```python
from build123d import *

# Parameters (mm, degrees)
SKETCH1_R           = 1.435
SKETCH1_R_2         = 1.4351
BOSS_EXTRUDE1_DEPTH = 3.175
SKETCH2_W           = 368.3
SKETCH2_H           = 127
CUT_EXTRUDE1_DEPTH  = 342.698968356
SKETCH4_R           = 1.89865
CUT_EXTRUDE2_DEPTH  = 342.698968356
SKETCH5_R           = 1.89865
CUT_EXTRUDE3_DEPTH  = 342.698968356


with BuildPart() as part:
    # Sketch1 → Boss-Extrude1 (new body)
    with BuildSketch(Plane.XY):
        with BuildLine():
            ThreePointArc((2.968751211, -181.189695026), (41.295889155, -181.079537948), (79.6220041, -180.778621425))
            Line((79.6220041, -180.778621425), (85.559165015, -180.714940362))
            ThreePointArc((85.559165015, -180.714940362), (123.887667874, -180.193645916), (162.213100977, -179.481566675))
            ThreePointArc((162.213100977, -179.481566675), (165.18118139, -179.418457741), (168.149237253, -179.35420455))
            ThreePointArc((168.149237253, -179.35420455), (192.659124698, -178.779845314), (217.167059321, -178.127456184))
            ThreePointArc((217.167059321, -178.127456184), (220.135246662, -178.043143258), (223.103401271, -177.957685792))
            Line((223.103401271, -177.957685792), (258.423629847, -176.852835003))
            ThreePointArc((258.423629847, -176.852835003), (267.290868319, -175.133004675), (275.18450496, -170.742533734))
            ThreePointArc((275.18450496, -170.742533734), (277.610750544, -168.6061656), (279.781359306, -166.210504095))
            ThreePointArc((279.781359306, -166.210504095), (284.283709644, -158.379432473), (286.129131597, -149.53685032))
            ThreePointArc((286.129131597, -149.53685032), (287.482131945, -117.828809116), (288.512976487, -86.108660213))
            ThreePointArc((288.512976487, -86.108660213), (288.592974065, -83.139049998), (288.670148028, -80.169365063))
            ThreePointArc((288.670148028, -80.169365063), (289.416235277, -41.572865854), (289.685382101, -2.970094485))
            ThreePointArc((289.685382101, -2.970094485), (289.686328933, 0.0005929), (289.684451162, 2.971279842))
            ThreePointArc((289.684451162, 2.971279842), (289.409759592, 41.084465923), (288.670148028, 79.191465063))
            ThreePointArc((288.670148028, 79.191465063), (288.592974065, 82.161149998), (288.512976487, 85.130760213))
            ThreePointArc((288.512976487, 85.130760213), (287.482131945, 116.850909116), (286.129131597, 148.55895032))
            ThreePointArc((286.129131597, 148.55895032), (284.283709644, 157.401532473), (279.781359306, 165.232604095))
            ThreePointArc((279.781359306, 165.232604095), (277.610750544, 167.6282656), (275.18450496, 169.764633734))
            ThreePointArc((275.18450496, 169.764633734), (267.290868319, 174.155104675), (258.423629847, 175.874935003))
            ThreePointArc((258.423629847, 175.874935003), (240.76414932, 176.447620699), (223.103401271, 176.979785792))
            ThreePointArc((223.103401271, 176.979785792), (220.135246662, 177.065243258), (217.167059321, 177.149556184))
            ThreePointArc((217.167059321, 177.149556184), (192.659124698, 177.801945314), (168.149237253, 178.37630455))
            ThreePointArc((168.149237253, 178.37630455), (165.18118139, 178.440557741), (162.213100977, 178.503666675))
            ThreePointArc((162.213100977, 178.503666675), (123.887667874, 179.215745916), (85.559165015, 179.737040362))
            ThreePointArc((85.559165015, 179.737040362), (82.590590695, 179.769453121), (79.6220041, 179.800721425))
            ThreePointArc((79.6220041, 179.800721425), (41.295889155, 180.101637948), (2.968751211, 180.211795026))
            ThreePointArc((2.968751211, 180.211795026), (0, 180.212367286), (-2.968751211, 180.211795026))
            ThreePointArc((-2.968751211, 180.211795026), (-41.295889155, 180.101637948), (-79.6220041, 179.800721425))
            ThreePointArc((-79.6220041, 179.800721425), (-82.590590695, 179.769453121), (-85.559165015, 179.737040362))
            ThreePointArc((-85.559165015, 179.737040362), (-123.887667874, 179.215745916), (-162.213100977, 178.503666675))
            ThreePointArc((-162.213100977, 178.503666675), (-165.18118139, 178.440557741), (-168.149237253, 178.37630455))
            ThreePointArc((-168.149237253, 178.37630455), (-192.659124698, 177.801945314), (-217.167059321, 177.149556184))
            ThreePointArc((-217.167059321, 177.149556184), (-220.135246662, 177.065243258), (-223.103401271, 176.979785792))
            ThreePointArc((-223.103401271, 176.979785792), (-240.76414932, 176.447620699), (-258.423629847, 175.874935003))
            ThreePointArc((-258.423629847, 175.874935003), (-267.290868319, 174.155104675), (-275.18450496, 169.764633734))
            ThreePointArc((-275.18450496, 169.764633734), (-277.610750544, 167.6282656), (-279.781359306, 165.232604095))
            ThreePointArc((-279.781359306, 165.232604095), (-284.283709644, 157.401532473), (-286.129131597, 148.55895032))
            ThreePointArc((-286.129131597, 148.55895032), (-287.482131945, 116.850909116), (-288.512976487, 85.130760213))
            ThreePointArc((-288.512976487, 85.130760213), (-288.592974065, 82.161149998), (-288.670148028, 79.191465063))
            ThreePointArc((-288.670148028, 79.191465063), (-289.409759592, 41.084465923), (-289.684451162, 2.971279842))
            ThreePointArc((-289.684451162, 2.971279842), (-289.686328933, 0.0005929), (-289.685382101, -2.970094485))
            ThreePointArc((-289.685382101, -2.970094485), (-289.416235277, -41.572865854), (-288.670148028, -80.169365063))
            ThreePointArc((-288.670148028, -80.169365063), (-288.592974065, -83.139049998), (-288.512976487, -86.108660213))
            ThreePointArc((-288.512976487, -86.108660213), (-287.482131945, -117.828809116), (-286.129131597, -149.53685032))
            ThreePointArc((-286.129131597, -149.53685032), (-284.283709644, -158.379432473), (-279.781359306, -166.210504095))
            ThreePointArc((-279.781359306, -166.210504095), (-277.610750544, -168.6061656), (-275.18450496, -170.742533734))
            ThreePointArc((-275.18450496, -170.742533734), (-267.290868319, -175.133004675), (-258.423629847, -176.852835003))
            ThreePointArc((-258.423629847, -176.852835003), (-240.76414932, -177.425520699), (-223.103401271, -177.957685792))
            ThreePointArc((-223.103401271, -177.957685792), (-220.135246662, -178.043143258), (-217.167059321, -178.127456184))
            ThreePointArc((-217.167059321, -178.127456184), (-192.659124698, -178.779845314), (-168.149237253, -179.35420455))
            ThreePointArc((-168.149237253, -179.35420455), (-165.18118139, -179.418457741), (-162.213100977, -179.481566675))
            ThreePointArc((-162.213100977, -179.481566675), (-123.887667874, -180.193645916), (-85.559165015, -180.714940362))
            ThreePointArc((-85.559165015, -180.714940362), (-82.590590695, -180.747353121), (-79.6220041, -180.778621425))
            ThreePointArc((-79.6220041, -180.778621425), (-41.295889155, -181.079537948), (-2.968751211, -181.189695026))
            ThreePointArc((-2.968751211, -181.189695026), (0, -181.190267286), (2.968751211, -181.189695026))
        make_face()
        with Locations((-274.954150451, -165.911566346)):
            Circle(SKETCH1_R, mode=Mode.SUBTRACT)
        with Locations((-220.027075225, -174.260724966)):
            Circle(SKETCH1_R_2, mode=Mode.SUBTRACT)
        with Locations((-165.1, -175.63472853)):
            Circle(SKETCH1_R_2, mode=Mode.SUBTRACT)
        with Locations((-82.55, -176.962970799)):
            Circle(SKETCH1_R_2, mode=Mode.SUBTRACT)
        with Locations((0, -177.405667286)):
            Circle(SKETCH1_R_2, mode=Mode.SUBTRACT)
        with Locations((-284.81033356, -83.03895)):
            Circle(SKETCH1_R_2, mode=Mode.SUBTRACT)
        with Locations((82.55, -176.962970799)):
            Circle(SKETCH1_R_2, mode=Mode.SUBTRACT)
        with Locations((165.1, -175.63472853)):
            Circle(SKETCH1_R_2, mode=Mode.SUBTRACT)
        with Locations((220.027075225, -174.260724966)):
            Circle(SKETCH1_R_2, mode=Mode.SUBTRACT)
        with Locations((274.954150451, -165.911566346)):
            Circle(SKETCH1_R_2, mode=Mode.SUBTRACT)
        with Locations((284.81033356, -83.03895)):
            Circle(SKETCH1_R_2, mode=Mode.SUBTRACT)
        with Locations((-285.902364234, 0)):
            Circle(SKETCH1_R_2, mode=Mode.SUBTRACT)
        with Locations((-284.81033356, 82.06105)):
            Circle(SKETCH1_R_2, mode=Mode.SUBTRACT)
        with Locations((-274.954150451, 164.933666346)):
            Circle(SKETCH1_R_2, mode=Mode.SUBTRACT)
        with Locations((-220.027075225, 173.282824966)):
            Circle(SKETCH1_R_2, mode=Mode.SUBTRACT)
        with Locations((-165.1, 174.65682853)):
            Circle(SKETCH1_R_2, mode=Mode.SUBTRACT)
        with Locations((-82.55, 175.985070799)):
            Circle(SKETCH1_R_2, mode=Mode.SUBTRACT)
        with Locations((0, 176.427767286)):
            Circle(SKETCH1_R_2, mode=Mode.SUBTRACT)
        with Locations((285.902364234, 0)):
            Circle(SKETCH1_R_2, mode=Mode.SUBTRACT)
        with Locations((284.81033356, 82.06105)):
            Circle(SKETCH1_R_2, mode=Mode.SUBTRACT)
        with Locations((82.55, 175.985070799)):
            Circle(SKETCH1_R_2, mode=Mode.SUBTRACT)
        with Locations((165.1, 174.65682853)):
            Circle(SKETCH1_R_2, mode=Mode.SUBTRACT)
        with Locations((220.027075225, 173.282824966)):
            Circle(SKETCH1_R_2, mode=Mode.SUBTRACT)
        with Locations((274.954150451, 164.933666346)):
            Circle(SKETCH1_R_2, mode=Mode.SUBTRACT)
    extrude(amount=BOSS_EXTRUDE1_DEPTH)

    # Sketch2 → Cut-Extrude1 (cut, through all)
    with BuildSketch(Plane.XY.offset(3.175)):
        with Locations((-76.579131597, 86.974935003)):
            Rectangle(SKETCH2_W, SKETCH2_H)
    extrude(amount=-CUT_EXTRUDE1_DEPTH, mode=Mode.SUBTRACT)

    # Sketch4 → Cut-Extrude2 (cut, through all)
    with BuildSketch(Plane(origin=(0, 0, 0), x_dir=(-1, 0, 0), z_dir=(0, 0, -1))):
        with Locations((-256.919131597, 144.124935003)):
            Circle(SKETCH4_R)
        with Locations((-132.419131597, 144.124935003)):
            Circle(SKETCH4_R)
        with Locations((-256.919131597, 19.624935003)):
            Circle(SKETCH4_R)
        with Locations((-256.919131597, 4.124935003)):
            Circle(SKETCH4_R)
        with Locations((-132.419131597, 19.624935003)):
            Circle(SKETCH4_R)
        with Locations((-132.419131597, 4.124935003)):
            Circle(SKETCH4_R)
        with Locations((-256.919131597, -120.375064997)):
            Circle(SKETCH4_R)
        with Locations((-132.419131597, -120.375064997)):
            Circle(SKETCH4_R)
    extrude(amount=-CUT_EXTRUDE2_DEPTH, mode=Mode.SUBTRACT)

    # Sketch5 → Cut-Extrude3 (cut, through all)
    with BuildSketch(Plane(origin=(0, 0, 0), x_dir=(-1, 0, 0), z_dir=(0, 0, -1))):
        with Locations((235.329131597, -145.102835003)):
            Circle(SKETCH5_R)
        with Locations((110.329131597, -145.102835003)):
            Circle(SKETCH5_R)
        with Locations((110.329131597, -20.102835003)):
            Circle(SKETCH5_R)
        with Locations((235.329131597, -20.102835003)):
            Circle(SKETCH5_R)
    extrude(amount=-CUT_EXTRUDE3_DEPTH, mode=Mode.SUBTRACT)


solid = part.part
```
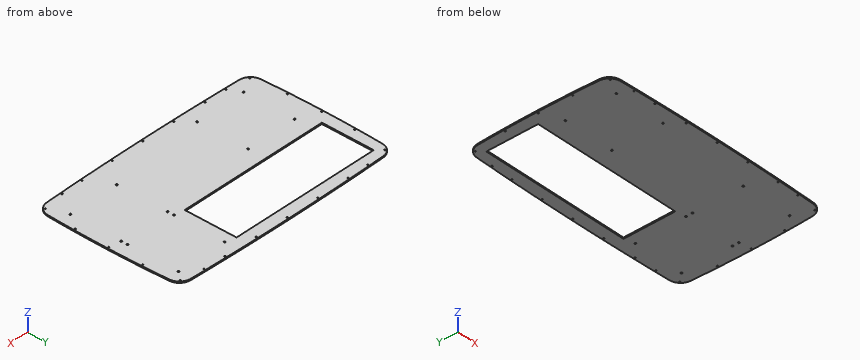
Check sheet for the modelled part. Datum: model origin and axes. Units: mm. Round coordinates to 2 decimals unless told otherwise and drop trailing zeros. Loops run counter-clockwise (first coordinate to the right, second up) from the corner with the lowest first, then second, coordinate; pieces in that order, holes last. Notation, with made-up numbers: (-9.75, -32) -> (13.25, -32) arc R17 ccw to (13.25, -9) -> close; hole circle Ø6 at (18, 4.25). An arc over 180 degrees is marked (long way). Answer in a Markdown table with one row per item.
Q1. Sectioned sample at D-D on x = 244. Enter the section's corners in (y, z) (3 decimals).
Data:
| item | result |
|---|---|
| outline | (-177.304, 0) -> (176.346, 0) -> (176.346, 3.175) -> (-177.304, 3.175) -> close |
Q2. Sectioned sample at C-C on z = 1. Give the number of separate pieces and of enclosed holes in the cut face, then the cut area to 3 significant figures.
Data:
| item | result |
|---|---|
| separate pieces | 1 |
| enclosed holes | 37 |
| area | 158,000 mm^2 |
Q3. Thickness scan on L1, parallel to Y at x = -88, z = 1.4; L2, parallel to Y at x = 91, z = 2.7; L3, parallel to X at y = 81.5, z = 1.65. Record the ranges inside material, lowest first.
Data:
| item | result |
|---|---|
| L1 | y = -180.69 to 23.47, 150.47 to 179.71 |
| L2 | y = -180.65 to 23.47, 150.47 to 179.67 |
| L3 | x = -288.61 to -286.13, -283.49 to -260.73, 107.57 to 283.49, 286.13 to 288.61 |
Q4. Sectioned sample at B-B on y = 64. Enter the section's corners in (x, z) (3 decimals).
Data:
| item | result |
|---|---|
| outline | (-289.021, 0) -> (-260.729, 0) -> (-260.729, 3.175) -> (-289.021, 3.175) -> close; (107.571, 0) -> (289.021, 0) -> (289.021, 3.175) -> (107.571, 3.175) -> close |
Q5. Sectioned sample at A-A on x = 46.5. Enter the section's corners in (y, z) (3 decimals), then the cut area to 3 significant figures.
Data:
| item | result |
|---|---|
| outline | (-181.05, 0) -> (23.475, 0) -> (23.475, 3.175) -> (-181.05, 3.175) -> close; (150.475, 0) -> (180.072, 0) -> (180.072, 3.175) -> (150.475, 3.175) -> close |
| area | 743 mm^2 |
Q6. Go/stop test with flat-tipped pins: P1, Ø3.5, axis at x = 165.1, y = 174.66, coming from the +Z side (3 decimals); P2, Ø2.5, axis at x = 274.95, y = -165.91, coming from the -Z side; P3, Ø1.5, axis at x = -141, z = 2.5, coming from the -Y side. Record where each tip stops, or that it passes through.
Data:
| item | result |
|---|---|
| P1 | stops at z = 3.175 |
| P2 | passes through |
| P3 | stops at y = -179.91 |
